The listing builds one solid part. Answer for the finished solid, in the listing's coordinates (mm). Face numbers are marked on the shaded views. A direction names the side the tool comes from. Coordinates: 2 decimals unless noted, no trailing zeros. Order: outer loops, then holes, each group sorted by start corner. A loop starts at its lowest first (then second) coordinate and runs counter-clockwise, first axis right, second up. Notation, with made-up numbers: (81, 36) -> (100, 36) arc R15 ccw to (100, 51) -> close; hole circle Ø5 at (-17, -27.75). An arc over 180 degrees is marked (long way). One line per question, with ' | ' between items.
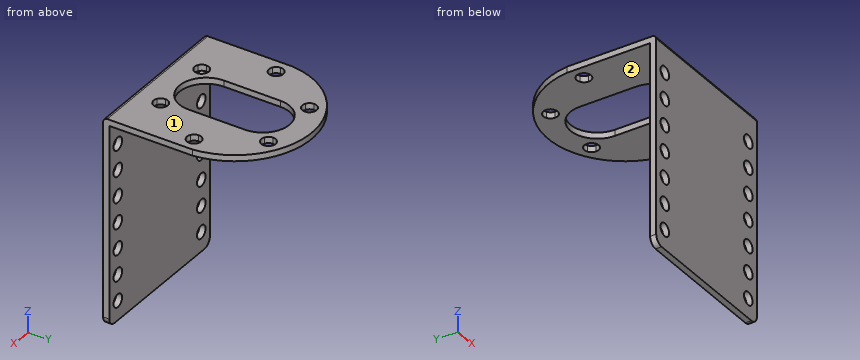
from build123d import *

# Parameters (mm, degrees)
BOSS_EXTRUDE1_DEPTH     = 1.5
SKETCH2_W               = 37.6
SKETCH2_H               = 50.8
BOSS_EXTRUDE2_DEPTH     = 1.5
FILLET1_R               = 1
FILLET2_R               = 2
SKETCH3_R               = 1.6
CUT_EXTRUDE1_DEPTH      = 1.5
LPATTERN1_COUNT         = 7
LPATTERN1_PITCH         = 6.4
MIRROR1_COPY_1_SKETCH_R = 1.6
MIRROR1_COPY_1_DEPTH    = 1.5
MIRROR1_COPY_2_SKETCH_R = 1.6
MIRROR1_COPY_2_DEPTH    = 1.5
MIRROR1_COPY_3_SKETCH_R = 1.6
MIRROR1_COPY_3_DEPTH    = 1.5
MIRROR1_COPY_4_SKETCH_R = 1.6
MIRROR1_COPY_4_DEPTH    = 1.5
MIRROR1_COPY_5_SKETCH_R = 1.6
MIRROR1_COPY_5_DEPTH    = 1.5
MIRROR1_COPY_6_SKETCH_R = 1.6
MIRROR1_COPY_6_DEPTH    = 1.5
SKETCH4_R               = 1.6
CUT_EXTRUDE2_DEPTH      = 1.5
CIRPATTERN1_COUNT       = 6


with BuildPart() as part:
    # Sketch1 → Boss-Extrude1 (new body)
    with BuildSketch(Plane.XY):
        with BuildLine():
            Line((-18.8, 0), (18.8, 0))
            Line((18.8, 0), (18.8, 22))
            ThreePointArc((18.8, 22), (0, 39), (-18.8, 22))
            Line((-18.8, 22), (-18.8, 0))
        make_face()
        with BuildLine():
            Line((-6.6, 12.999434154), (-6.6, 26.899434154))
            ThreePointArc((-6.6, 26.899434154), (0, 33.5), (6.6, 26.899434154))
            Line((6.6, 26.899434154), (6.6, 12.999434154))
            ThreePointArc((6.6, 12.999434154), (0, 6.399999946), (-6.6, 12.999434154))
        make_face(mode=Mode.SUBTRACT)
    extrude(amount=BOSS_EXTRUDE1_DEPTH)

    # Sketch2 → Boss-Extrude2 (add)
    with BuildSketch(Plane.XZ):
        with Locations((0, -23.9)):
            Rectangle(SKETCH2_W, SKETCH2_H)
    extrude(amount=-BOSS_EXTRUDE2_DEPTH)

    # Fillet1
    fillet1_edges = [part.edges().sort_by_distance(p)[0] for p in [
        (0, 0, 1.5),
    ]]
    fillet(fillet1_edges, radius=FILLET1_R)

    # Fillet2
    fillet2_edges = [part.edges().sort_by_distance(p)[0] for p in [
        (-18.8, 0.75, -49.3),
        (18.8, 0.75, -49.3),
    ]]
    fillet(fillet2_edges, radius=FILLET2_R)

    # Sketch3 → Cut-Extrude1 (cut)
    with BuildSketch(Plane.XZ):
        with Locations((-15.6, -44.5)):
            Circle(SKETCH3_R)
    cut_extrude1 = extrude(amount=-CUT_EXTRUDE1_DEPTH, mode=Mode.SUBTRACT)

    # LPattern1: Cut-Extrude1 ×7
    with Locations(*[(0, 0, i * LPATTERN1_PITCH) for i in range(1, LPATTERN1_COUNT)]):
        add(cut_extrude1, mode=Mode.SUBTRACT)

    # Mirror1: Cut-Extrude1 across plane
    add(cut_extrude1.mirror(Plane(origin=(0, 0, 0), x_dir=(0, 0, 1), z_dir=(1, 0, 0))), mode=Mode.SUBTRACT)

    # Mirror1 copy 1 sketch → Mirror1 copy 1 (cut)
    with BuildSketch(Plane(origin=(0, 0, 6.4), x_dir=(-1, 0, 0), z_dir=(0, -1, 0))):
        with Locations((-15.6, 44.5)):
            Circle(MIRROR1_COPY_1_SKETCH_R)
    extrude(amount=-MIRROR1_COPY_1_DEPTH, mode=Mode.SUBTRACT)

    # Mirror1 copy 2 sketch → Mirror1 copy 2 (cut)
    with BuildSketch(Plane(origin=(0, 0, 12.8), x_dir=(-1, 0, 0), z_dir=(0, -1, 0))):
        with Locations((-15.6, 44.5)):
            Circle(MIRROR1_COPY_2_SKETCH_R)
    extrude(amount=-MIRROR1_COPY_2_DEPTH, mode=Mode.SUBTRACT)

    # Mirror1 copy 3 sketch → Mirror1 copy 3 (cut)
    with BuildSketch(Plane(origin=(0, 0, 19.2), x_dir=(-1, 0, 0), z_dir=(0, -1, 0))):
        with Locations((-15.6, 44.5)):
            Circle(MIRROR1_COPY_3_SKETCH_R)
    extrude(amount=-MIRROR1_COPY_3_DEPTH, mode=Mode.SUBTRACT)

    # Mirror1 copy 4 sketch → Mirror1 copy 4 (cut)
    with BuildSketch(Plane(origin=(0, 0, 25.6), x_dir=(-1, 0, 0), z_dir=(0, -1, 0))):
        with Locations((-15.6, 44.5)):
            Circle(MIRROR1_COPY_4_SKETCH_R)
    extrude(amount=-MIRROR1_COPY_4_DEPTH, mode=Mode.SUBTRACT)

    # Mirror1 copy 5 sketch → Mirror1 copy 5 (cut)
    with BuildSketch(Plane(origin=(0, 0, 32), x_dir=(-1, 0, 0), z_dir=(0, -1, 0))):
        with Locations((-15.6, 44.5)):
            Circle(MIRROR1_COPY_5_SKETCH_R)
    extrude(amount=-MIRROR1_COPY_5_DEPTH, mode=Mode.SUBTRACT)

    # Mirror1 copy 6 sketch → Mirror1 copy 6 (cut)
    with BuildSketch(Plane(origin=(0, 0, 38.4), x_dir=(-1, 0, 0), z_dir=(0, -1, 0))):
        with Locations((-15.6, 44.5)):
            Circle(MIRROR1_COPY_6_SKETCH_R)
    extrude(amount=-MIRROR1_COPY_6_DEPTH, mode=Mode.SUBTRACT)

    # Sketch4 → Cut-Extrude2 (cut)
    with BuildSketch(Plane.XY.offset(1.5)):
        with Locations((7.664771385, 33.22577344)):
            Circle(SKETCH4_R)
        with Locations((15.32954277, 19.949999973)):
            Circle(SKETCH4_R)
        with Locations((7.664771385, 6.674226506)):
            Circle(SKETCH4_R)
        with Locations((-7.664771385, 6.674226506)):
            Circle(SKETCH4_R)
        with Locations((-15.32954277, 19.949999973)):
            Circle(SKETCH4_R)
        with Locations((-7.664771385, 33.22577344)):
            Circle(SKETCH4_R)
    cut_extrude2 = extrude(amount=-CUT_EXTRUDE2_DEPTH, mode=Mode.SUBTRACT)

    # CirPattern1: Cut-Extrude2 ×6 about axis
    cirpattern1_axis = Axis((0, 20.104705882, 0), (0, 0, 1))
    for i in range(1, CIRPATTERN1_COUNT):
        add(cut_extrude2.rotate(cirpattern1_axis, i * 360 / CIRPATTERN1_COUNT), mode=Mode.SUBTRACT)


solid = part.part
Item 1: Section C-C, the plane x = 0 is taken. Give the vertices of the cut face in (y, z).
Computed values:
outline: (0, -49.3) -> (1.5, -49.3) -> (1.5, 0) -> (6.4, 0) -> (6.4, 1.5) -> (1, 1.5) arc R1 ccw to (0, 0.5) -> close; (33.5, 0) -> (39, 0) -> (39, 1.5) -> (33.5, 1.5) -> close
Item 2: Section A-A, the plane y = 15.5 is taken. Give the vertices of the cut face in (x, z), plus the area to 3 significant figures.
Computed values:
outline: (-18.8, 0) -> (-6.6, 0) -> (-6.6, 1.5) -> (-18.8, 1.5) -> close; (6.6, 0) -> (18.8, 0) -> (18.8, 1.5) -> (6.6, 1.5) -> close | area: 36.6 mm^2
Item 3: For the marked faces 1 and 2, determine the directions among +Z, -Z, +X, -X, +Y, -Y from which every point of the face is accessible in a straight line to the end or side of a thin tool.
Computed values:
face 1: +Z, +X, -X, +Y, -Y | face 2: -Z, +X, -X, +Y
Item 4: This flat-tipped pin is pushed along its axis until it touches: pin 1 Ø8 at (x, z) = (6, -28.5) entering from +Y. Where does it stop, or does it pass through?
Computed values:
pin 1: stops at y = 1.5
Item 5: Find the intervals of material crossed by L1, parallel to Y at x = 8, z = -14.5, in increasing order.
Computed values:
L1: y = 0 to 1.5
Item 6: Section B-B, the plane z = -12.5 is taken. Give the vertices of the cut face in (x, y).
Computed values:
outline: (-18.8, 0) -> (-17.2, 0) -> (-17.2, 1.5) -> (-18.8, 1.5) -> close; (-14, 0) -> (14, 0) -> (14, 1.5) -> (-14, 1.5) -> close; (17.2, 0) -> (18.8, 0) -> (18.8, 1.5) -> (17.2, 1.5) -> close
Item 7: Section D-D, the plane x = -11.5 is taken. Give the vertices of the cut face in (y, z), plus the area to 3 significant figures.
Computed values:
outline: (0, -49.3) -> (1.5, -49.3) -> (1.5, 0) -> (35.1, 0) -> (35.1, 1.5) -> (1, 1.5) arc R1 ccw to (0, 0.5) -> close | area: 126 mm^2
